from build123d import *

# Parameters (mm, degrees)
F0_R     = 44
F0_R_2   = 11.325
F1_DEPTH = 7
F2_R     = 3.5
F3_R     = 3.49999


# Not quite as in the source:
# - a fillet or chamfer is up to 0.001 mm smaller than in the source, because OpenCascade refuses the exact size


with BuildPart() as f1:
    # F0 (on Top) → F1 (new body)
    with BuildSketch(Plane.XY):
        Circle(F0_R)
        with Locations((-23.0534838522, -13.3099351078)):
            Circle(F0_R_2, mode=Mode.SUBTRACT)
        with Locations((0, -26.6198702157)):
            Circle(F0_R_2, mode=Mode.SUBTRACT)
        with Locations((23.0534838522, -13.3099351078)):
            Circle(F0_R_2, mode=Mode.SUBTRACT)
        with Locations((-23.0534838522, 13.3099351078)):
            Circle(F0_R_2, mode=Mode.SUBTRACT)
        Circle(F0_R_2, mode=Mode.SUBTRACT)
        with Locations((23.0534838522, 13.3099351078)):
            Circle(F0_R_2, mode=Mode.SUBTRACT)
        with Locations((0, 26.6198702157)):
            Circle(F0_R_2, mode=Mode.SUBTRACT)
    extrude(amount=F1_DEPTH)

    # F2
    f2_edges = [f1.edges().sort_by_distance(p)[0] for p in [
        (-44, 0, 7),
    ]]
    fillet(f2_edges, radius=F2_R)

    # F3 (radius 3.5 in the source; OpenCascade refuses exactly that, so slightly less here)
    f3_edges = [f1.edges().sort_by_distance(p)[0] for p in [
        (-44, 0, 0),
    ]]
    fillet(f3_edges, radius=F3_R)


solid = f1.part
Verification items for the finished model (mm, model axes). Coordinates: 2 decimals unless noted, no trailing zeros. Write each loop counter-clockwise with the first axis right and the second up, starting at its lowest first coordinate (ties: lowest second). Pieces come first, ordered by that corner, then holes. Notation, with made-up numbers: (40, 51) - (72, 51) arc R27 ccw to (72, 79) - close; hole circle Ø4 at (2, 50). An arc over 180 degrees is marked (long way). Answer as a JSON object with one key per item and string values.
(1) Thickness scan on line 1 along Y through (x, z) = (16.5, 4.75); line 2 along Y through (x, z) = (-24, 0.5); line 3 along X through (y, z) = (-19, 6). Record the ranges inside material, lowest first.
Report:
{"line 1": "-40.54 to -22.55, -4.07 to 4.07, 22.55 to 40.54", "line 2": "-34.84 to -24.6, -2.02 to 2.02, 24.6 to 34.84", "line 3": "-38.52 to -32.85, -13.26 to -8.38, 8.38 to 13.26, 32.85 to 38.52"}
(2) Cross-section at C-C on z = 5.25. Record the cut outline in (x, y) (3 decimals).
Report:
{"outline": "circle Ø87.062 at (0, 0); hole circle Ø22.65 at (-23.053, -13.31); hole circle Ø22.65 at (-23.053, 13.31); hole circle Ø22.65 at (0, -26.62); hole circle Ø22.65 at (0, 0); hole circle Ø22.65 at (0, 26.62); hole circle Ø22.65 at (23.053, -13.31); hole circle Ø22.65 at (23.053, 13.31)"}
(3) Cross-section at A-A on x = 0. Give the number of separate pieces and of enclosed holes in the cut face, plus the area to 3 significant figures.
Report:
{"separate pieces": "4", "enclosed holes": "0", "area": "130 mm^2"}
(4) Mould release check, pull along Y, two halves, no side actions. Record for faces 1 (the cylindrical face through (-2.455, -11.056, 3.451)), 2 (the flat face through (8.4, -8.4, 7)): pulls with the +Y half, pulls with the -Y half, needs draft (parallel to the pull), parting line crosses it, or undercut.
Report:
{"face 1": "undercut", "face 2": "needs draft"}
(5) Gauge pin test, flat ends, axial feed: pin 1 Ø13.5 at (x, y) = (0, -26.62) entering from +Z; pin 2 Ø1 at (x, z) = (-6, 5) entering from -Y; pin 3 Ø1.5 at (y, z) = (-16, 2) entering from +X. Record the tip position at first contact, or that the pin passes through.
Report:
{"pin 1": "through", "pin 2": "y = -43.46", "pin 3": "x = 41.05"}
